```python
from build123d import *

# Parameters (mm, degrees)
CYLINDER009_R     = 1.7
CYLINDER009_DEPTH = 30
CYLINDER007_R     = 1.7
CYLINDER007_DEPTH = 30
BOX015_W          = 25.4
BOX015_H          = 8
BOX015_DEPTH      = 2


with BuildPart() as cylinder009:
    # Cylinder009 → Cylinder009 (new body)
    with BuildSketch(Plane(origin=(128, 46.8, -127), x_dir=(1, 0, 0), z_dir=(0, 0, 1))):
        Circle(CYLINDER009_R)
    extrude(amount=CYLINDER009_DEPTH)


with BuildPart() as cylinder007:
    # Cylinder007 → Cylinder007 (new body)
    with BuildSketch(Plane(origin=(111, 46.8, -127), x_dir=(1, 0, 0), z_dir=(0, 0, 1))):
        Circle(CYLINDER007_R)
    extrude(amount=CYLINDER007_DEPTH)


with BuildPart() as cut010:
    # Box015 → Box015 (new body)
    with BuildSketch(Plane(origin=(106.8, 42.8, -110), x_dir=(1, 0, 0), z_dir=(0, 0, 1))):
        with Locations((12.7, 4)):
            Rectangle(BOX015_W, BOX015_H)
    extrude(amount=BOX015_DEPTH)

    # Cut009: cut Cylinder007
    add(cylinder007.part, mode=Mode.SUBTRACT)

    # Cut010: cut Cylinder009
    add(cylinder009.part, mode=Mode.SUBTRACT)


solid = cut010.part
```
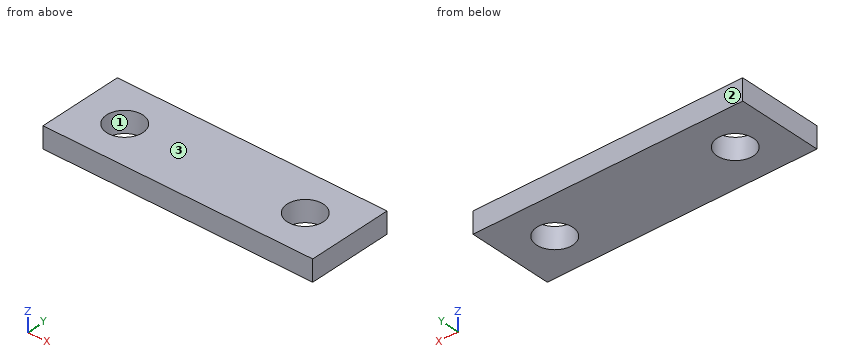
CAD build for the part. Positions are in the model's coordinates, mm. Face numbers are marked on the shaded views. Coordinates: 2 decimals unless noted, no trailing zeros. Write each loop counter-clockwise with the first axis right and the second up, starting at its lowest first coordinate (ties: lowest second). Pieces come first, ordered by that corner, then holes.
(1) Drill centre lines: probe 1 along X at (y, z) = (46.8, -108.55); probe 2 along Y at (x, z) = (111, -109.4); probe 3 along X at (y, z) = (46.25, -108.5). Where is each one in solid material? Low to high.
(2) Cut at B-B, the plane z = -108.95. List the corners of the cut face in (x, y), and give its area (3 significant figures).
(3) Two-plate mould, pull along Y, no slides. Class the marked faces 1, 2 and 3: +Y half, -Y half, draft (parallel to the pull), parting line (faces both ways), or undercut.
(4) Cut at A-A, the plane y = 46.8. List the corners of the cut face in (x, z).
(5) Cut at C-C, the plane x = 128. List the corners of the cut face in (y, z).
(6) Flat gauge pin, fed straight in: pin 1 (2 mm diameter, centred on x = 111, y = 46.8, fed in from -Z). Where does the tip first touch, or does it go through?
Geometry says:
1. probe 1: x = 106.8 to 109.3, 112.7 to 126.3, 129.7 to 132.2
1. probe 2: y = 42.8 to 45.1, 48.5 to 50.8
1. probe 3: x = 106.8 to 109.39, 112.61 to 126.39, 129.61 to 132.2
2. outline: (106.8, 42.8) - (132.2, 42.8) - (132.2, 50.8) - (106.8, 50.8) - close; hole circle Ø3.4 at (111, 46.8); hole circle Ø3.4 at (128, 46.8)
2. area: 185 mm2
3. face 1: undercut
3. face 2: +Y half
3. face 3: draft
4. outline: (106.8, -110) - (109.3, -110) - (109.3, -108) - (106.8, -108) - close; (112.7, -110) - (126.3, -110) - (126.3, -108) - (112.7, -108) - close; (129.7, -110) - (132.2, -110) - (132.2, -108) - (129.7, -108) - close
5. outline: (42.8, -110) - (45.1, -110) - (45.1, -108) - (42.8, -108) - close; (48.5, -110) - (50.8, -110) - (50.8, -108) - (48.5, -108) - close
6. pin 1: passes through
